The figure shows three views and two pictorial views of one solid part (mm, origin at its lowest corner). Answer the questions. Round coordinates to 2 decimals unless told otherwise and drop trailing zeros. Order: outer loops, then holes, each group sorted by start corner. A loop starts at its lowest first (then second) coordinate and runs counter-clockwise, first axis right, second up. Notation, with made-up numbers: (49.5, 49) -> (63.5, 49) arc R7 cw to (63.5, 59) -> close; hole circle Ø10 at (87.5, 13). An arc over 180 degrees is marked (long way). Answer as a JSON object with one key per item and string values. Group by question number.
Item 1: Given P1, Ø2, axis at x = 29.5, z = 18, coming from the -Y side; P2, Ø1.5, axis at y = 1.5, z = 18, coming from the +X side; P3, Ø1.1, axis at x = 11.5, y = 1.5, coming from the +Z side (3 decimals), each flat-ended and moving along its own axis, determine where each tip first touches the part or whether it passes through.
Item 2: Consider probe 1 along X at (y, z) = (3, 20); probe 2 along Y at (x, z) = (51.5, 8); probe 3 along X at (y, z) = (5, 32) (1 decimal). Determine where each line is inside the solid, lowest interval first. Write a range as from..to.
Item 3: Section B-B, the plane y = 2 is taken. Write down the section's boundary in (x, z) (1 decimal), plus the area to 3 significant figures.
Item 4: Section A-A, the plane x = 11.5 is taken. Write down the section's boundary in (y, z) (1 decimal).
Item 5: Section C-C, the plane z = 12.5 is taken. Write down the section's boundary in (x, y), plus the area to 3 significant figures.
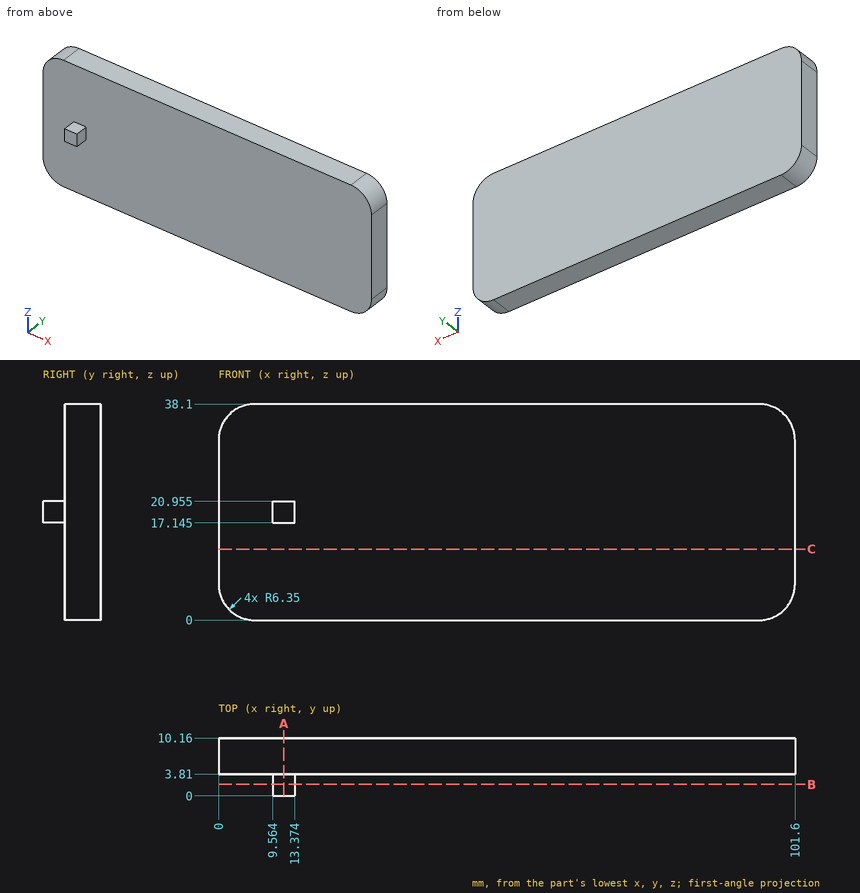
Values found:
{
 "1": {"P1": "y = 3.81", "P2": "x = 13.37", "P3": "z = 20.955"},
 "2": {"probe 1": "9.56..13.37", "probe 2": "3.81..10.16", "probe 3": "0..101.6"},
 "3": {"outline": "(9.6, 17.1) -> (13.4, 17.1) -> (13.4, 21) -> (9.6, 21) -> close", "area": "14.5 mm2"},
 "4": {"outline": "(0, 17.1) -> (3.8, 17.1) -> (3.8, 0) -> (10.2, 0) -> (10.2, 38.1) -> (3.8, 38.1) -> (3.8, 21) -> (0, 21) -> close"},
 "5": {"outline": "(0, 3.81) -> (101.6, 3.81) -> (101.6, 10.16) -> (0, 10.16) -> close", "area": "645 mm2"}
}
